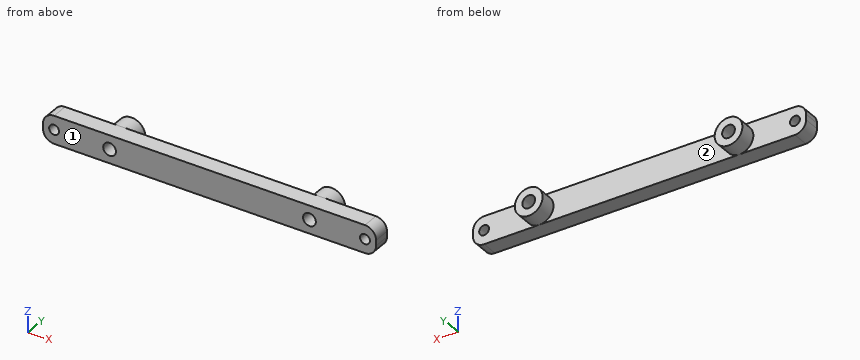
Autodesk Inventor part; units mm, degrees
ref_plane "YZ Plane" through (0, 0, 0) normal (1, 0, 0) x (0, 1, 0)
ref_plane "XZ Plane" through (0, 0, 0) normal (0, 1, 0) x (-1, 0, 0)
ref_plane "XY Plane" through (0, 0, 0) normal (0, 0, 1) x (1, 0, 0)
sketch "Sketch1" plane through (0, 0, 0) normal (0, 1, 0) x (-1, 0, 0)
  line L0 (30, -2.5) -> (-30, -2.5)
  line L1 (-30, -2.5) -> (-30, 2.5)
  line L2 (-30, 2.5) -> (30, 2.5)
  line L3 (30, 2.5) -> (30, -2.5)
  line L4 (30, -2.5) -> (-30, 2.5) construction
  line L5 (-30, -2.5) -> (30, 2.5) construction
  point P0 (0, 0)
  dimension "d0" = 60
  dimension "d1" = 5
extrude "Extrusion1" add sketch "Sketch1" along normal blind 3
sketch "Sketch2" plane through (0, 3, 0) normal (0, 1, 0) x (1, 0, 0)
  line L0 (-30, -2.5) -> (30, -2.5)
  line L1 (30, -2.5) -> (30, 2.5)
  line L2 (30, 2.5) -> (-30, 2.5)
  line L3 (-30, 2.5) -> (-30, -2.5)
  line L4 (-30, 2.5) -> (30, -2.5) construction
  line L5 (30, 2.5) -> (-30, -2.5) construction
  line L6 (-30, 0) -> (30, 0) construction
  line L7 (0, 2.5) -> (0, -2.5) construction
  circle A0 centre (-18, 0) radius 2.5
  circle A1 centre (18, 0) radius 2.5
  point P0 (0, 0)
  dimension "d4" = 5
  dimension "d5" = 18
extrude "Extrusion2" add sketch "Sketch2" along normal blind 3 contours A0 | A1
sketch "Sketch3" plane through (-18, 6, 0) normal (0, 1, 0) x (1, 0, 0)
  circle A0 centre (0, 0) radius 2.5
  circle A1 centre (36, 0) radius 2.5
  point P0 (18, 0)
hole "Hole1" at (-18, 6, 0) at (18, 6, 0) direction (0, -1, 0) diameter 2.3 end through all
fillet "Fillet1" radius 2 4 edges at (-30, 1.5, -2.5) (-30, 1.5, 2.5) (30, 1.5, -2.5) (30, 1.5, 2.5)
sketch "Sketch4" plane through (0, 3, 0) normal (0, 1, 0) x (1, 0, 0)
  arc A0 (28, -2.5) -> (30, -0.5) centre (28, -0.5) ccw
  line L0 (30, -0.5) -> (30, 0.5)
  arc A1 (30, 0.5) -> (28, 2.5) centre (28, 0.5) ccw
  line L1 (28, 2.5) -> (18, 2.5)
  arc A2 (-28, 2.5) -> (-30, 0.5) centre (-28, 0.5) ccw
  line L2 (-30, 0.5) -> (-30, -0.5)
  arc A3 (-30, -0.5) -> (-28, -2.5) centre (-28, -0.5) ccw
  line L3 (-28, -2.5) -> (-18, -2.5)
  arc A4 (18, -2.5) -> (18, 2.5) centre (18, 0) ccw
  arc A5 (-18, -2.5) -> (-18, 2.5) centre (-18, 0) ccw
  line L4 (-30, 0) -> (30, 0) construction
  line L5 (-28, 0.5) -> (-28, -0.5) construction
  line L6 (28, 0.5) -> (28, -0.5) construction
  arc A6 (18, 2.5) -> (18, -2.5) centre (18, 0) ccw
  line L7 (18, 2.5) -> (-18, 2.5)
  line L8 (-18, -2.5) -> (18, -2.5)
  arc A7 (-18, 2.5) -> (-18, -2.5) centre (-18, 0) ccw
  line L9 (-18, 2.5) -> (-28, 2.5)
  line L10 (18, -2.5) -> (28, -2.5)
  point P0 (0, 0)
  point P1 (-28, 0)
  point P2 (28, 0)
hole "Hole2" at (-28, 3, 0) at (28, 3, 0) direction (0, -1, 0) diameter 1.778 end through all
properties part number "Busbar Base"
Input: part model. Units: mm. Frame: model coordinates. Face numbers are marked on the shaded views. Give positions to 0.01 mm unless a question says otherwise; leave off trailing zeros. Order: outer loops, then holes, each group sorted by start corner. A loop starts at its lowest first (then second) coordinate and runs counter-clockwise, first axis right, second up.
1. Material intervals for L1, parallel to X at y = 3.2, z = 0; L2, parallel to X at y = 1.9, z = 0; L3, parallel to Z at x = 28, y = 2.3, sorted ascending.
Derived:
L1: x = -20.5 to -19.15, -16.85 to -15.5, 15.5 to 16.85, 19.15 to 20.5
L2: x = -30 to -28.89, -27.11 to -19.15, -16.85 to 16.85, 19.15 to 27.11, 28.89 to 30
L3: z = -2.5 to -0.89, 0.89 to 2.5
2. Section A-A on y = 2.2. Return the cut outline in (x, z), and give its area (3 significant figures).
Derived:
outline: (-30, -0.5) arc R2 ccw to (-28, -2.5) - (28, -2.5) arc R2 ccw to (30, -0.5) - (30, 0.5) arc R2 ccw to (28, 2.5) - (-28, 2.5) arc R2 ccw to (-30, 0.5) - close; hole circle Ø1.78 at (-28, 0); hole circle Ø2.3 at (-18, 0); hole circle Ø2.3 at (18, 0); hole circle Ø1.78 at (28, 0)
area: 283 mm2
3. Section D-D on z = -1.8. Return the cut outline in (x, y).
Derived:
outline: (-29.52, 0) - (29.52, 0) - (29.52, 3) - (19.73, 3) - (19.73, 6) - (16.27, 6) - (16.27, 3) - (-16.27, 3) - (-16.27, 6) - (-19.73, 6) - (-19.73, 3) - (-29.52, 3) - close
4. Section B-B on x = 18.5. Return the cut outline in (y, z), and give its area (3 significant figures).
Derived:
outline: (0, -2.5) - (3, -2.5) - (3, -2.45) - (6, -2.45) - (6, -1.04) - (0, -1.04) - close; (0, 1.04) - (6, 1.04) - (6, 2.45) - (3, 2.45) - (3, 2.5) - (0, 2.5) - close
area: 17.3 mm2
5. Section C-C on y = 5.1. Return the cut outline in (x, z).
Derived:
outline: circle Ø5 at (-18, 0); circle Ø5 at (18, 0); hole circle Ø2.3 at (-18, 0); hole circle Ø2.3 at (18, 0)
6. Pin query (flat end, axial travel): pin 1 (3 mm diameter, centred on x = -28, z = 0, fed in from +Y); pin 2 (1.8 mm diameter, centred on x = -18, z = 0, fed in from +Y). Return the tip coordinate at first contact, or that it passes through.
Derived:
pin 1: stops at y = 3
pin 2: passes through
7. Mould query, pull axis X, two halves, no side actions, for the marked faces 1 and 2. Classes: released by +X, released by -X, zero draft, split by the parting line, or undercut.
Derived:
face 1: zero draft
face 2: undercut
